Could you check a few things on this model? Use its own coordinates, in mm. A direction names the side the tool comes from. Give positions to 0.01 mm unless a question says otherwise; leave off trailing zeros. Loops run counter-clockwise (first coordinate to the right, second up) from the corner with the lowest first, then second, coordinate; pieces in that order, holes last. Notation, with made-up numbers: M 88,-40 L 109,-40 A27 cw 109,-17 Z; hole C 77,87 d9. An arc over 180 degrees is marked long. Answer in a Markdown table with one row per item. Add a question column.
1. I'm going to push flat-ended pins straight in: pin 1 Ø9 at (x, z) = (6.5, 0) entering from +Y; pin 2 Ø3 at (y, z) = (4.5, -10) entering from +X; pin 3 Ø8 at (x, y) = (5, 12) entering from -Z; pin 4 Ø2 at (x, y) = (-4, 6) entering from -Z. Where does each tip first touch, or does it pass through?
2. If we section it at D-D on y = 8: List the corners of the cut face in (x, z) for me.
3. If we section it at A-A on z = 0: List the corners of the cut face in (x, y) for me.
4. If we section it at B-B on x = 0: List the corners of the cut face in (y, z) for me, then the cut area to 3 significant figures.
5. If we section it at C-C on z = 11.5: List the corners of the cut face in (x, y) for me.
6. I need wall thicknesses on line 1 along X through (y, z) = (7.25, 0); line 2 along Y through (x, z) = (-1, 12); line 3 along X through (y, z) = (13, 0). Which ranges of each line are inside material? Lowest first, please. Write a range as from..to.
7. Which directions (+Z, -Z, +X, -X, +Y, -Y) give clear straight access to the entire face, cutting with the end or side of a thin tool? Please do faces 5 (the flat face through (0, 8, 1)), 6 (the cylindrical face through (-3.905, 13.972, -0.867)), 7 (the cylindrical face through (0, 6, 10)).
8. Thinking about a two-plate mould opening in Y: for faces 1 (the flat face through (0, 16, 2)), 2 (the flat face through (3, 0, 0)), 3 (the flat face through (10, 1.5, 3)), 4 (the flat face through (10, 10.5, -3)), which applies, released by +Y, released by -Y, zero draft, split by the parting line, or undercut?
```python
from build123d import *

# Parameters (mm, degrees)
SKETCH2_R           = 4
BOSS_EXTRUDE1_DEPTH = 4
CUT_EXTRUDE1_DEPTH  = 16
SKETCH4_R           = 0.75
CUT_EXTRUDE2_DEPTH  = 16


with BuildPart() as part:
    # Sketch1 → Revolve1 (revolve)
    with BuildSketch(Plane.XY, mode=Mode.PRIVATE) as revolve1_sk:
        Polygon((0, 0), (0, 12), (15, 12), (15, 10.5), (10, 10.5), (10, 1.5), (15, 1.5), (15, 0), align=None)
    revolve(revolve1_sk.sketch.rotate(Axis((0, 0, 0), (0, 1, 0)), 90), axis=Axis((0, 0, 0), (0, 1, 0)))

    # Sketch2 → Boss-Extrude1 (add)
    with BuildSketch(Plane(origin=(0, 12, 0), x_dir=(1, 0, 0), z_dir=(0, 1, 0))):
        with Locations(Location((0, 0, 0), (0, 0, 270))):
            Circle(SKETCH2_R)
    extrude(amount=BOSS_EXTRUDE1_DEPTH)

    # Sketch3 → Cut-Extrude1 (cut)
    with BuildSketch(Plane.XZ):
        with BuildLine():
            Line((-1.184271928, 1), (1.184271928, 1))
            ThreePointArc((1.184271928, 1), (0, -1.55), (-1.184271928, 1))
        make_face()
    extrude(amount=-CUT_EXTRUDE1_DEPTH, mode=Mode.SUBTRACT)

    # Sketch4 → Cut-Extrude2 (cut)
    with BuildSketch(Plane.XZ):
        with Locations(Location((0, 11.5, 0), (0, 0, 270))):
            Circle(SKETCH4_R)
    extrude(amount=-CUT_EXTRUDE2_DEPTH, mode=Mode.SUBTRACT)


solid = part.part
```
Results:
| question | item | result |
|---|---|---|
| 1 | pin 1 | y = 16 |
| 1 | pin 2 | x = 5.27 |
| 1 | pin 3 | z = -14.97 |
| 1 | pin 4 | z = -9.54 |
| 2 | outline | C 0,0 d20; hole M -1.18,1 A1.55 ccw long 1.18,1 Z |
| 3 | outline | M -15,0 L -1.55,0 L -1.55,16 L -4,16 L -4,12 L -15,12 L -15,10.5 L -10,10.5 L -10,1.5 L -15,1.5 Z; M 1.55,0 L 15,0 L 15,1.5 L 10,1.5 L 10,10.5 L 15,10.5 L 15,12 L 4,12 L 4,16 L 1.55,16 Z |
| 4 | outline | M 0,-15 L 1.5,-15 L 1.5,-10 L 10.5,-10 L 10.5,-15 L 12,-15 L 12,-4 L 16,-4 L 16,-1.55 L 0,-1.55 Z; M 0,1 L 16,1 L 16,4 L 12,4 L 12,10.75 L 10.5,10.75 L 10.5,10 L 1.5,10 L 1.5,10.75 L 0,10.75 Z; M 0,12.25 L 1.5,12.25 L 1.5,15 L 0,15 Z; M 10.5,12.25 L 12,12.25 L 12,15 L 10.5,15 Z |
| 4 | area | 257 mm2 |
| 5 | outline | M -9.63,0 L -0.75,0 L -0.75,1.5 L -9.63,1.5 Z; M -9.63,10.5 L -0.75,10.5 L -0.75,12 L -9.63,12 Z; M 0.75,0 L 9.63,0 L 9.63,1.5 L 0.75,1.5 Z; M 0.75,10.5 L 9.63,10.5 L 9.63,12 L 0.75,12 Z |
| 6 | line 1 | -10..-1.55, 1.55..10 |
| 6 | line 2 | 0..1.5, 10.5..12 |
| 6 | line 3 | -4..-1.55, 1.55..4 |
| 7 | face 5 | +Y, -Y |
| 7 | face 6 | +Y |
| 7 | face 7 | none |
| 8 | face 1 | released by +Y |
| 8 | face 2 | released by -Y |
| 8 | face 3 | undercut |
| 8 | face 4 | undercut |
